Input: part model. Units: mm. Frame: model coordinates. Round coordinates to 2 decimals unless told otherwise and drop trailing zeros. Order: outer loops, then holes, each group sorted by start corner. A loop starts at its lowest first (then second) coordinate and runs counter-clockwise, first axis right, second up.
Item 1: Cut plane D-D on z = 5.5. Output: boundary loops of the cut face in (x, y).
Item 2: Line query: L1, parallel to Y at x = 0, z = 3.85; L2, parallel to Y at x = 0.35, z = 3.25; L3, parallel to Z at x = -0.3, y = -1.25. Output: solid intervals per line, ascending.
Item 3: Cut plane A-A on y = -0.75. Output: boundary loops of the cut face in (x, z).
Item 4: Cut plane B-B on z = 3.5. Output: boundary loops of the cut face in (x, y).
Item 5: Cut plane C-C on x = 0.05. Output: boundary loops of the cut face in (y, z) (3 decimals), then the cut area to 3 significant figures.
```python
from build123d import *

# Parameters (mm, degrees)
BOSS_EXTRUDE1_DEPTH      = 0.5
BOSS_EXTRUDE1_DEPTH_BACK = 0.5
SKETCH1_R                = 0.85


with BuildPart() as part:
    # Sketch1 → Boss-Extrude1 (new, two sides: drawn at the far end of the back side and taken through both)
    with BuildSketch(Plane(origin=(0, 0, 0), x_dir=(0, 0, -1), z_dir=(1, 0, 0)).offset(-BOSS_EXTRUDE1_DEPTH_BACK)):
        with BuildLine():
            Line((-2.173337586, -6.105456882), (-2.107128968, -5.919460069))
            ThreePointArc((-2.107128968, -5.919460069), (-2.517494945, -4.015728705), (-4.40445692, -3.534098298))
            ThreePointArc((-4.40445692, -3.534098298), (-5.854874371, -3.387705714), (-6.748960786, -2.23629308))
            ThreePointArc((-6.748960786, -2.23629308), (0, 6.5), (6.748960786, -2.23629308))
            ThreePointArc((6.748960786, -2.23629308), (5.854874409, -3.387705693), (4.404457002, -3.534098324))
            ThreePointArc((4.404457002, -3.534098324), (2.517494975, -4.015728674), (2.107128968, -5.919460069))
            Line((2.107128968, -5.919460069), (2.173337586, -6.105456882))
            ThreePointArc((2.173337586, -6.105456882), (3.247964263, -7.151631133), (4.732703867, -6.939849718))
            ThreePointArc((4.732703867, -6.939849718), (0, 8.4), (-4.732703867, -6.939849718))
            ThreePointArc((-4.732703867, -6.939849718), (-3.247964263, -7.151631133), (-2.173337586, -6.105456882))
        make_face()
        with Locations((3.85, -5.29905652)):
            Circle(SKETCH1_R, mode=Mode.SUBTRACT)
        with Locations((-3.85, -5.29905652)):
            Circle(SKETCH1_R, mode=Mode.SUBTRACT)
    extrude(amount=BOSS_EXTRUDE1_DEPTH + BOSS_EXTRUDE1_DEPTH_BACK)


solid = part.part
```
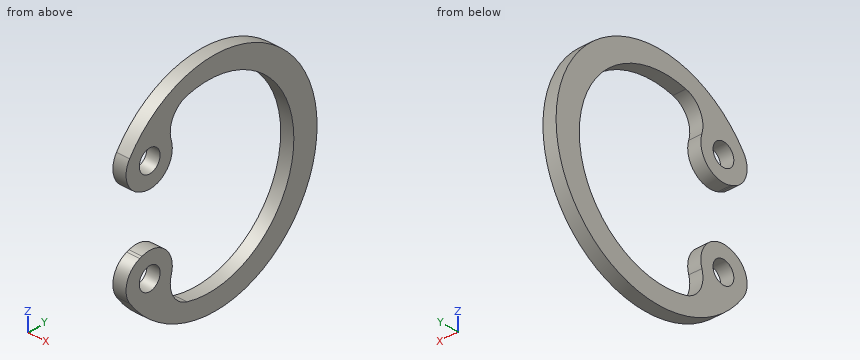
From the geometry:
1. outline: (-0.5, -6.35) - (0.5, -6.35) - (0.5, -3.54) - (-0.5, -3.54) - close; (-0.5, 3.81) - (0.5, 3.81) - (0.5, 6.35) - (-0.5, 6.35) - close
2. L1: y = -7.23 to -6.15, -4.45 to -3.45, 5.34 to 7.47
2. L2: y = -7.15 to -5.9, -4.7 to -3.55, 5.7 to 7.75
2. L3: z = -8.31 to -6.93, 6.93 to 8.31
3. outline: (-0.5, -8.37) - (0.5, -8.37) - (0.5, -6.97) - (-0.5, -6.97) - close; (-0.5, 6.97) - (0.5, 6.97) - (0.5, 8.37) - (-0.5, 8.37) - close
4. outline: (-0.5, -7.21) - (0.5, -7.21) - (0.5, -6.07) - (-0.5, -6.07) - close; (-0.5, -4.52) - (0.5, -4.52) - (0.5, -3.48) - (-0.5, -3.48) - close; (-0.5, 5.56) - (0.5, 5.56) - (0.5, 7.64) - (-0.5, 7.64) - close
5. outline: (-6.94, -4.733) arc R8.4 ccw (long way) to (-6.94, 4.733) arc R1.7 ccw to (-6.105, 2.173) - (-5.919, 2.107) arc R1.85 ccw to (-3.534, 4.404) arc R1.85 cw to (-2.236, 6.749) arc R6.975 cw (long way) to (-2.236, -6.749) arc R1.85 cw to (-3.534, -4.404) arc R1.85 ccw to (-5.919, -2.107) - (-6.105, -2.173) arc R1.7 ccw to start; hole circle Ø1.7 at (-5.299, -3.85); hole circle Ø1.7 at (-5.299, 3.85)
5. area: 75.7 mm2
